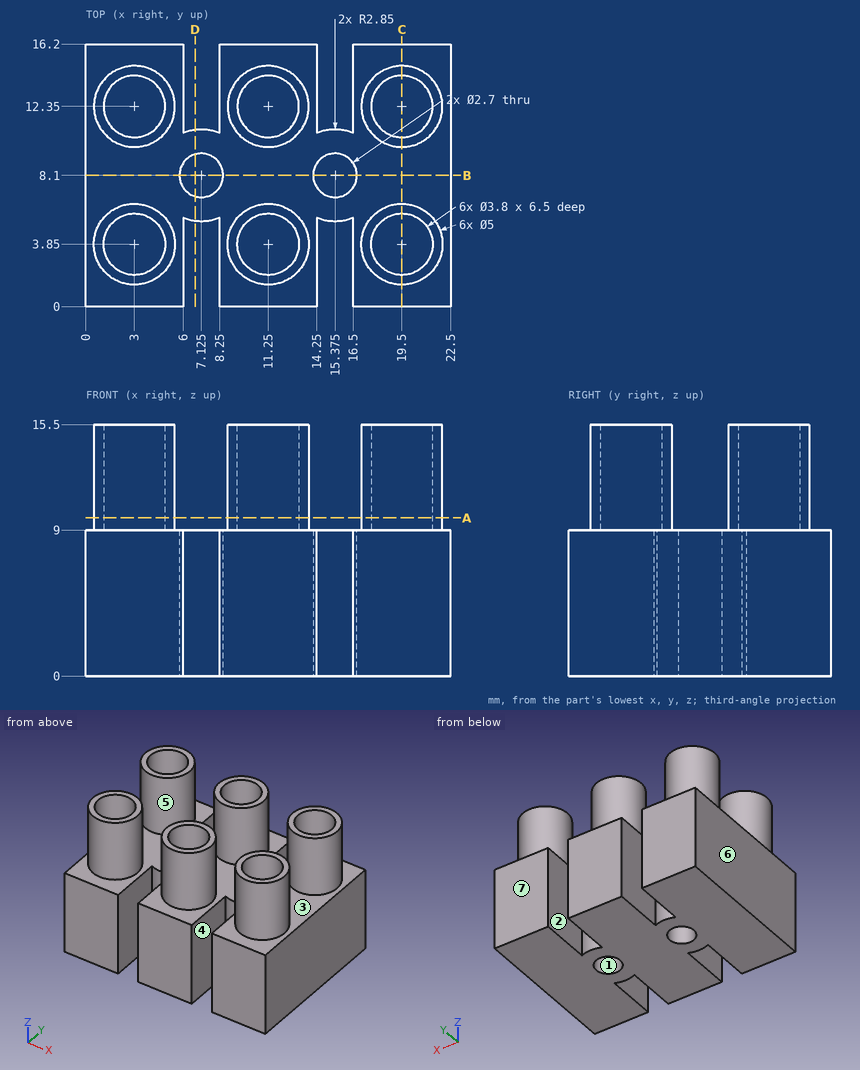
Geometry: see drawing. Coordinates: mm, zero at the bounding-box minimum. A direction names the side the tool comes from. Give positions to 0.01 mm unless a question says otherwise; leave off trailing zeros. Write each loop counter-clockwise with the first axis right and the second up, starting at its lowest first coordinate (ties: lowest second). Pieces come first, ordered by that corner, then holes. Notation, with made-up numbers: M -27,59 L 29,59 A15 ccw 29,75 Z; hole C -23,55 d7. An arc over 180 degrees is marked long. Return JSON: item names as keys, results as strings. Group by question number.
1) Ray query, L1, parallel to X at y = 3, z = 5.5; L2, parallel to X at y = 5.5, z = 11.25; L3, parallel to Y at x = 7.25, z = 3.25. Return the intervals inside material, ascending.
2) Cut plane B-B, the plane y = 8.1. Output: boundary loops of the cut face in (x, z) (3 decimals), then the cut area to 3 significant figures.
3) First-contact query: pin 1 Ø1 at (x, y) = (9.5, 12) entering from +Z; pin 2 Ø1 at (x, y) = (19.5, 13.5) entering from +Z; pin 3 Ø3 at (y, z) = (2, 12) entering from +X; pin 4 Ø1.6 at (x, y) = (15.375, 8.1) entering from -Z. Flat tips, straight axial feed; report the tip coordinate or a pass-through.
4) Cut plane C-C, the plane x = 19.5. Output: boundary loops of the cut face in (y, z).
5) Draft query along X for the marked faces 5, 6 and 7. Return one class per face: released by +X, released by -X, zero draft, split by the parting line, or undercut.
6) Cut plane D-D, the plane x = 6.75. Output: boundary loops of the cut face in (y, z), then the cut area to 3 significant figures.
7) Cut plane A-A, the plane z = 9.75. Give the number of separate pieces and of enclosed holes in the cut face, then the cut area to 3 significant figures.
8) Set-up query: the marked faces 1, 2, 3 and 4. Return all of +Z, -Z, +X, -X, +Y, -Y with unobstructed straight access to the full face (end or side cutting, diameter ignored); none if empty.
Data:
{
 "1": {"L1": "x = 0 to 6, 8.25 to 14.25, 16.5 to 22.5", "L2": "x = 1.12 to 2.06, 3.94 to 4.88, 9.37 to 10.31, 12.19 to 13.13, 17.62 to 18.56, 20.44 to 21.38", "L3": "y = 5.25 to 6.76, 9.44 to 10.95"},
 "2": {"outline": "M 0,0 L 5.775,0 L 5.775,9 L 0,9 Z; M 8.475,0 L 14.025,0 L 14.025,9 L 8.475,9 Z; M 16.725,0 L 22.5,0 L 22.5,9 L 16.725,9 Z", "area": "154 mm²"},
 "3": {"pin 1": "stops at z = 15.5", "pin 2": "stops at z = 9", "pin 3": "stops at x = 21.98", "pin 4": "passes through"},
 "4": {"outline": "M 0,0 L 16.2,0 L 16.2,9 L 14.85,9 L 14.85,15.5 L 14.25,15.5 L 14.25,9 L 10.45,9 L 10.45,15.5 L 9.85,15.5 L 9.85,9 L 6.35,9 L 6.35,15.5 L 5.75,15.5 L 5.75,9 L 1.95,9 L 1.95,15.5 L 1.35,15.5 L 1.35,9 L 0,9 Z"},
 "5": {"face 5": "undercut", "face 6": "released by -X", "face 7": "zero draft"},
 "6": {"outline": "M 5.27,0 L 6.8,0 L 6.8,9 L 5.27,9 Z; M 9.4,0 L 10.93,0 L 10.93,9 L 9.4,9 Z", "area": "27.5 mm²"},
 "7": {"separate pieces": "6", "enclosed holes": "6", "area": "49.8 mm²"},
 "8": {"face 1": "+Z, -Z", "face 2": "+Z, -Z, +Y", "face 3": "+Z", "face 4": "+Z, -Z, -Y"}
}
